from build123d import *

# Parameters (mm, degrees)
SKETCH1_R           = 80
BOSS_EXTRUDE1_DEPTH = 40
SKETCH2_R           = 60
CUT_EXTRUDE1_DEPTH  = 17
SKETCH3_R           = 25
CUT_EXTRUDE2_DEPTH  = 24
SKETCH4_R           = 3
CUT_EXTRUDE3_DEPTH  = 24
SKETCH6_R           = 60
CUT_EXTRUDE4_DEPTH  = 17
SKETCH7_R           = 65
CUT_EXTRUDE5_DEPTH  = 1
SKETCH8_R           = 65
CUT_EXTRUDE6_DEPTH  = 1
FILLET1_R           = 15
FILLET2_R           = 15


with BuildPart() as part:
    # Sketch1 → Boss-Extrude1 (new body)
    with BuildSketch(Plane(origin=(0, 0, 0), x_dir=(1, 0, 0), z_dir=(0, 1, 0))):
        Circle(SKETCH1_R)
    extrude(amount=BOSS_EXTRUDE1_DEPTH)

    # Sketch2 → Cut-Extrude1 (cut)
    with BuildSketch(Plane(origin=(0, 40, 0), x_dir=(1, 0, 0), z_dir=(0, 1, 0))):
        Circle(SKETCH2_R)
    extrude(amount=-CUT_EXTRUDE1_DEPTH, mode=Mode.SUBTRACT)

    # Sketch3 → Cut-Extrude2 (cut, through all)
    with BuildSketch(Plane(origin=(0, 23, 0), x_dir=(1, 0, 0), z_dir=(0, 1, 0))):
        Circle(SKETCH3_R)
    extrude(amount=-CUT_EXTRUDE2_DEPTH, mode=Mode.SUBTRACT)

    # Sketch4 → Cut-Extrude3 (cut, through all)
    with BuildSketch(Plane(origin=(0, 23, 0), x_dir=(1, 0, 0), z_dir=(0, 1, 0))):
        with Locations((0, 35)):
            Circle(SKETCH4_R)
        with Locations((30.310889132, 17.5)):
            Circle(SKETCH4_R)
        with Locations((30.310889132, -17.5)):
            Circle(SKETCH4_R)
        with Locations((0, -35)):
            Circle(SKETCH4_R)
        with Locations((-30.310889132, -17.5)):
            Circle(SKETCH4_R)
        with Locations((-30.310889132, 17.5)):
            Circle(SKETCH4_R)
    extrude(amount=-CUT_EXTRUDE3_DEPTH, mode=Mode.SUBTRACT)

    # Sketch6 → Cut-Extrude4 (cut)
    with BuildSketch(Plane.XZ):
        Circle(SKETCH6_R)
    extrude(amount=-CUT_EXTRUDE4_DEPTH, mode=Mode.SUBTRACT)

    # Sketch7 → Cut-Extrude5 (cut)
    with BuildSketch(Plane.XZ):
        Circle(SKETCH7_R)
    extrude(amount=-CUT_EXTRUDE5_DEPTH, mode=Mode.SUBTRACT)

    # Sketch8 → Cut-Extrude6 (cut)
    with BuildSketch(Plane(origin=(0, 40, 0), x_dir=(1, 0, 0), z_dir=(0, 1, 0))):
        Circle(SKETCH8_R)
    extrude(amount=-CUT_EXTRUDE6_DEPTH, mode=Mode.SUBTRACT)

    # Fillet1
    fillet1_edges = [part.edges().sort_by_distance(p)[0] for p in [
        (-60, 23, 0),
    ]]
    fillet(fillet1_edges, radius=FILLET1_R)

    # Fillet2
    fillet2_edges = [part.edges().sort_by_distance(p)[0] for p in [
        (-60, 17, 0),
    ]]
    fillet(fillet2_edges, radius=FILLET2_R)


solid = part.part
Verification items for the finished model (mm, model axes). A direction names the side the tool comes from. Coordinates: 2 decimals unless noted, no trailing zeros. Order: outer loops, then holes, each group sorted by start corner. A loop starts at its lowest first (then second) coordinate and runs counter-clockwise, first axis right, second up.
Item 1: Section check C-C, the plane y = 7.5. Enter the section's corners in (x, z).
Filled in:
outline: circle Ø160 at (0, 0); hole circle Ø117.91 at (0, 0)
Item 2: Material ranges on L1, parallel to Z at x = 0, y = 20.65; L2, parallel to X at y = 20, z = -17; L3, parallel to X at y = 20.5, z = -17.5, recorded low to high.
Filled in:
L1: z = -80 to -38, -32 to -25, 25 to 32, 38 to 80
L2: x = -78.17 to -33.27, -27.35 to -18.33, 18.33 to 27.35, 33.27 to 78.17
L3: x = -78.06 to -33.31, -27.31 to -17.85, 17.85 to 27.31, 33.31 to 78.06
Item 3: Release check for a two-part mould opening along Z. For faces 4 (the face through (19, 1, -57.5)), 5 (the face through (0, 0, -66)), 6 (the face through (-17.34, 19.72, 78.1)) record: +Z half, -Z half, draft (parallel to the pull), parting line (faces both ways), or undercut.
Filled in:
face 4: undercut
face 5: draft
face 6: parting line
Item 4: Access from +Z, -Z, +X, -X, +Y, -Y to the whole of each face (thin tool, end or side, straight path). Record for faces 1 (the face through (19, 23, 19)), 2 (the face through (19, 17, -19)), 3 (the face through (23.846, 20.042, -7.509)).
Filled in:
face 1: +Y
face 2: -Y
face 3: +Y, -Y
Item 5: Section check A-A, the plane z = 0. Enter the section's corners in (x, y), then the cut area to 3 significant figures.
Filled in:
outline: (-80, 0) - (-65, 0) - (-65, 1) - (-60, 1) - (-60, 2) arc R15 cw to (-45, 17) - (-25, 17) - (-25, 23) - (-45, 23) arc R15 cw to (-60, 38) - (-60, 39) - (-65, 39) - (-65, 40) - (-80, 40) - close; (25, 17) - (45, 17) arc R15 cw to (60, 2) - (60, 1) - (65, 1) - (65, 0) - (80, 0) - (80, 40) - (65, 40) - (65, 39) - (60, 39) - (60, 38) arc R15 cw to (45, 23) - (25, 23) - close
area: 2,190 mm2
Item 6: Depth check by flat-ended pin: pin 1 (3 mm diameter, centred on x = -37, z = -5, fed in from +Y); pin 2 (12 mm diameter, centred on y = 11, z = 34, fed in from -X); pin 3 (12 mm diameter, centred on y = 17, z = -34.5, fed in from +X). Enter the tip coordinate at first touch or a pass-through.
Filled in:
pin 1: stops at y = 23
pin 2: stops at x = -74.94
pin 3: stops at x = 74.75
Item 7: Section check B-B, the plane x = 0. Give the number of separate pieces and of enclosed holes in the cut face, then the cut area to 3 significant figures.
Filled in:
separate pieces: 4
enclosed holes: 0
area: 2,120 mm2
